Here's the drawing with two shaded views (mm, measured from the low corner). I have some questions. A direction names the side the tool comes from. Round coordinates to 2 decimals unless told otherwise and drop trailing zeros. Write each loop counter-clockwise with the first axis right and the second up, starting at its lowest first coordinate (ties: lowest second). Pieces come first, ordered by that corner, then holes. Notation, with made-up numbers: M 70,-26 L 97,-26 A25 ccw 97,-11 Z; hole C -3.5,17.5 d11. An arc over 180 degrees is marked long. Answer as a JSON object with one key per item and string values. Group by question number.
1) Suppose I cut it at A-A, the plane z = 8.5. Write out the boundary of the cut face in (x, y).
2) Please list where these lines run through material, in increasing order: L1, parallel to Z at x = 4.95, y = 2.5; L2, parallel to Y at x = 2.85, z = 2.5; L3, parallel to Y at x = 3.65, z = 3.5 (1 decimal). Write a range as [from, to].
3) I'm going to push flat-ended pins straight in: pin 1 Ø2 at (x, z) = (3, 5) entering from -Y (1 decimal); pin 2 Ø1 at (x, y) = (1.5, 5) entering from -Z. Where does each tip first touch, or does it pass through?
4) On a 3-axis mill with a long thin cutter (end or side, diameter ignored), from which of +Z, -Z, +X, -X, +Y, -Y can I reach the whole of each face in a straight line? I mean the marked faces 1 and 2. Say none if no direction works.
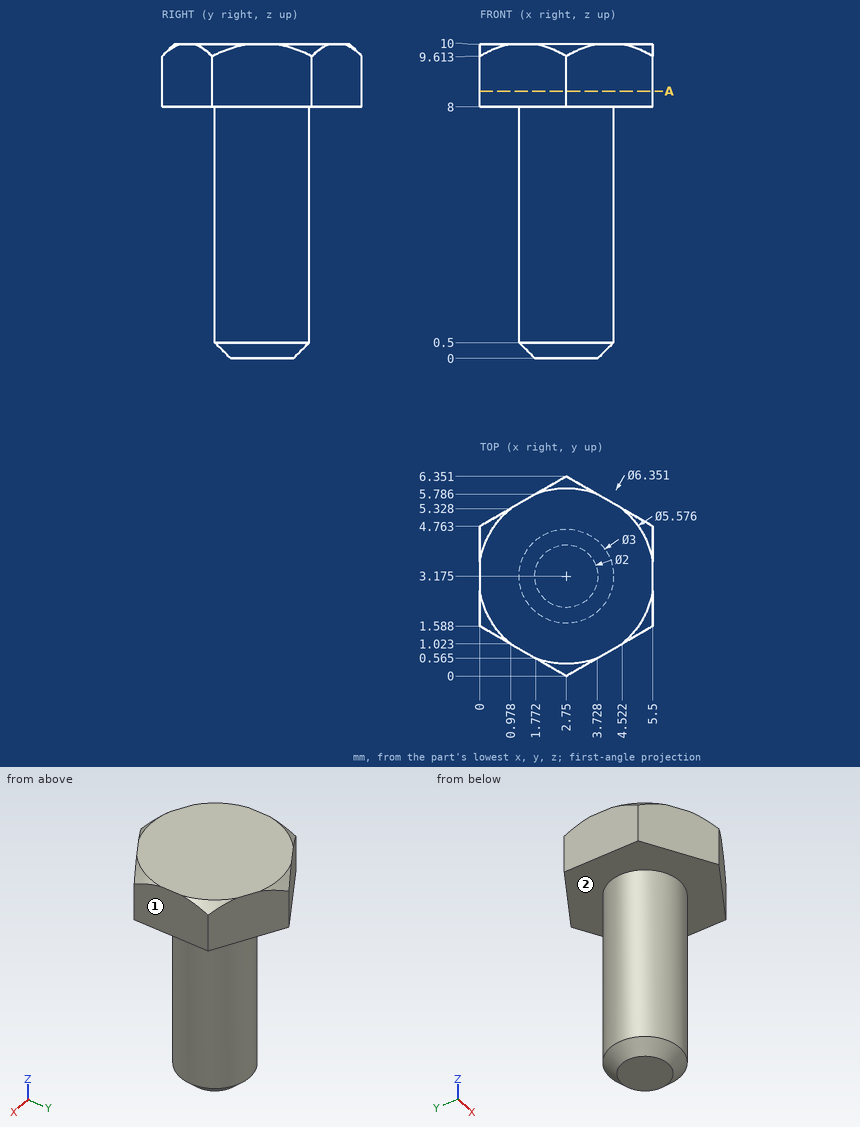
Results:
{
 "1": {"outline": "M 0,1.59 L 2.75,0 L 5.5,1.59 L 5.5,4.76 L 2.75,6.35 L 0,4.76 Z"},
 "2": {"L1": "[8, 10]", "L2": "[1.68, 4.67]", "L3": "[2, 4.4]"},
 "3": {"pin 1": "y = 1.7", "pin 2": "z = 8"},
 "4": {"face 1": "+Z, -Z, +X, +Y, -Y", "face 2": "-Z"}
}
